from build123d import *

# Parameters (mm, degrees)
CBORE_SOCKET_HEAD_CAP_SCREW1_D           = 4.5
CBORE_SOCKET_HEAD_CAP_SCREW1_CBORE_D     = 8
CBORE_SOCKET_HEAD_CAP_SCREW1_CBORE_DEPTH = 4.1
DELETEFACE1_START                        = 17
DELETEFACE1_OUTLINE_R                    = 4
DELETEFACE1_DEPTH                        = 8
CUT_EXTRUDE2_DEPTH                       = 38.32961291
CBORE_SOCKET_HEAD_CAP_SCREW2_D           = 4.5
CBORE_SOCKET_HEAD_CAP_SCREW2_CBORE_D     = 8
CBORE_SOCKET_HEAD_CAP_SCREW2_CBORE_DEPTH = 4.1


# Read off the part's stored shape, not the designer's step: DeleteFace1
with BuildPart() as part:
    # Sketch1 → Revolve1 (revolve)
    with BuildSketch(Plane.XY, mode=Mode.PRIVATE) as revolve1_sk:
        Polygon((25, 12), (25, 23.5), (17, 23.5), (17, 15), (0, 15), (0, 12), (1.5, 12), (1.5, 12.6), (2.85, 12.6), (2.85, 12), (7.85, 12), (7.85, 10), (17.15, 10), (17.15, 12), (22.15, 12), (22.15, 12.6), (23.5, 12.6), (23.5, 12), align=None)
    revolve(revolve1_sk.sketch.rotate(Axis((25, 0, 0), (-1, 0, 0)), 90), axis=Axis((25, 0, 0), (-1, 0, 0)))

    # CBORE Socket Head Cap Screw1 (through all)
    with Locations(Plane(origin=(25, 0, 0), x_dir=(0, 0, -1), z_dir=(1, 0, 0))):
        with Locations((0, 18.5), (18.5, 0), (-18.5, 0), (0, -18.5)):
            CounterBoreHole(CBORE_SOCKET_HEAD_CAP_SCREW1_D / 2, CBORE_SOCKET_HEAD_CAP_SCREW1_CBORE_D / 2, CBORE_SOCKET_HEAD_CAP_SCREW1_CBORE_DEPTH)

    # DeleteFace1 outline → DeleteFace1 (add)
    with BuildSketch(Plane.YZ.offset(DELETEFACE1_START)):
        with Locations((-18.5, 0)):
            Circle(DELETEFACE1_OUTLINE_R)
        with Locations((0, 18.5)):
            Circle(DELETEFACE1_OUTLINE_R)
        with Locations((0, -18.5)):
            Circle(DELETEFACE1_OUTLINE_R)
        with Locations((18.5, 0)):
            Circle(DELETEFACE1_OUTLINE_R)
    extrude(amount=DELETEFACE1_DEPTH)

    # Sketch5 → Cut-Extrude2 (cut, through all)
    with BuildSketch(Plane(origin=(17, 0, 0), x_dir=(0, 0, -1), z_dir=(1, 0, 0))):
        with BuildLine():
            Line((-16, 17.211914478), (-16, -17.211914478))
            ThreePointArc((-16, -17.211914478), (-23.5, 0), (-16, 17.211914478))
        make_face()
        with BuildLine():
            Line((16, 17.211914478), (16, -17.211914478))
            ThreePointArc((16, -17.211914478), (23.5, 0), (16, 17.211914478))
        make_face()
    extrude(amount=CUT_EXTRUDE2_DEPTH, mode=Mode.SUBTRACT)

    # CBORE Socket Head Cap Screw2 (through all)
    with Locations(Plane(origin=(25, 0, 0), x_dir=(0, 0, -1), z_dir=(1, 0, 0))):
        with Locations((0, 18.5), (0, -18.5)):
            CounterBoreHole(CBORE_SOCKET_HEAD_CAP_SCREW2_D / 2, CBORE_SOCKET_HEAD_CAP_SCREW2_CBORE_D / 2, CBORE_SOCKET_HEAD_CAP_SCREW2_CBORE_DEPTH)


solid = part.part
Part model, mm, in its own coordinate system. A direction names the side the tool comes from. Coordinates: 2 decimals unless noted, no trailing zeros. Order: outer loops, then holes, each group sorted by start corner. A loop starts at its lowest first (then second) coordinate and runs counter-clockwise, first axis right, second up. Notation, with made-up numbers: M 22,-23.5 L 61,-23.5 A32 ccw 61,12.5 Z; hole C -9.5,75.5 d5. An arc over 180 degrees is marked long. Use a Markdown table: item, result.
(1) Flat gauge pins, fed straight in: pin 1 (2 mm diameter, centred on y = -6.5, z = -4, fed in from -X); pin 2 (6.5 mm diameter, centred on y = 17.5, z = 1, fed in from +X); pin 3 (5 mm diameter, centred on x = 12.5, z = -4.5, fed in from -Y); pin 4 (4 mm diameter, centred on x = 9.5, y = -6.5, fed in from +Z). Where does each tip first touch, or does it go through?
A:
| item | result |
|---|---|
| pin 1 | passes through |
| pin 2 | stops at x = 25 |
| pin 3 | stops at y = -14.87 |
| pin 4 | stops at z = 14.31 |
(2) Pull direction Y, two halves, no side cores. Call faces 1 (the cylindrical face through (8.38, -12.65, -8.06)), 2 (the cylindrical face through (22.979, 22.466, 0.521)), 3 (the cylindrical face through (22.979, -14.534, 0.521)), 4 (the flat face through (21, 0, 16)): released by +Y, released by -Y, zero draft, split by the parting line, or undercut.
A:
| item | result |
|---|---|
| face 1 | split by the parting line |
| face 2 | undercut |
| face 3 | undercut |
| face 4 | zero draft |
(3) Cut at C-C on x = 5.5. Write the cut outline in (y, z), then the cut area to 3 significant figures.
A:
| item | result |
|---|---|
| outline | C 0,0 d30; hole C 0,0 d24 |
| area | 254 mm^2 |
(4) Cut at D-D on z = 0. State how many separate pieces and enclosed holes the cut face has, then the cut area to 3 significant figures.
A:
| item | result |
|---|---|
| separate pieces | 4 |
| enclosed holes | 0 |
| area | 219 mm^2 |
(5) Tool access for faces 5 (the cylindrical face through (22.834, 7.667, 9.999)), 6 (the cylindrical face through (5.385, -3.604, -11.446)), 7 (the cylindrical face through (24.26, -3.604, -11.446)): list every direction of +Z, -Z, +X, -X, +Y, -Y with a clear straight run to the whole face (end or side of a thin tool).
A:
| item | result |
|---|---|
| face 5 | none |
| face 6 | -X |
| face 7 | +X |
(6) Cut at B-B on y = 13.5. Write the cut outline in (x, z).
A:
| item | result |
|---|---|
| outline | M 0,-6.54 L 17,-6.54 L 17,-16 L 25,-16 L 25,16 L 17,16 L 17,6.54 L 0,6.54 Z |
(7) Cut at A-A on y = 18.5. Write the cut outline in (x, z), then the cut area to 3 significant figures.
A:
| item | result |
|---|---|
| outline | M 17,-14.49 L 25,-14.49 L 25,-4 L 20.9,-4 L 20.9,-2.25 L 17,-2.25 Z; M 17,2.25 L 20.9,2.25 L 20.9,4 L 25,4 L 25,14.49 L 17,14.49 Z |
| area | 182 mm^2 |
(8) Probe L1, parallel to Y at x = 18.45, z = 0; L2, parallel to Y at x = 23.35, z = 0; L3, parallel to Z at x = 23.75, y = 7. List the from-to ranges inside material, lowest first.
A:
| item | result |
|---|---|
| L1 | y = -23.5 to -20.75, -16.25 to -12, 12 to 16.25, 20.75 to 23.5 |
| L2 | y = -23.5 to -22.5, -14.5 to -12.6, 12.6 to 14.5, 22.5 to 23.5 |
| L3 | z = -16 to -9.75, 9.75 to 16 |
